from build123d import *

# Parameters (mm, degrees)
BOSS_EXTRUDE1_DEPTH = 1
SKETCH2_R           = 1
SKETCH2_W           = 7
SKETCH2_H           = 23.92041254
SKETCH2_H_2         = 5
BOSS_EXTRUDE4_DEPTH = 29
BOSS_EXTRUDE5_DEPTH = 7
SKETCH2_4_R         = 1
CUT_EXTRUDE1_DEPTH  = 29
CUT_EXTRUDE2_REACH  = 70.069
SKETCH5_W           = 7
SKETCH5_H           = 2


with BuildPart() as part:
    # Sketch1 → Boss-Extrude1 (new body)
    with BuildSketch(Plane(origin=(0, 0, 0), x_dir=(1, 0, 0), z_dir=(0, 1, 0))):
        Polygon((46.188021535, 0), (23.094010768, 40), (-23.094010768, 40), (-46.188021535, 0), (-23.094010768, -40), (23.094010768, -40), align=None)
    extrude(amount=BOSS_EXTRUDE1_DEPTH)

    # Sketch2 → Boss-Extrude4 (add)
    # profile 1 of 5: a face of its own
    with BuildSketch(Plane(origin=(0, 1, 0), x_dir=(1, 0, 0), z_dir=(0, 1, 0))):
        with Locations(Location((-14.1, -4.8, 0), (0, 0, 90))):
            Circle(SKETCH2_R)
    # profile 2 of 5: a face of its own
    with BuildSketch(Plane(origin=(0, 1, 0), x_dir=(1, 0, 0), z_dir=(0, 1, 0))):
        with Locations(Location((-14.1, 4.8, 0), (0, 0, 90))):
            Circle(SKETCH2_R)
    # profile 3 of 5: a face of its own
    with BuildSketch(Plane(origin=(0, 1, 0), x_dir=(1, 0, 0), z_dir=(0, 1, 0))):
        with Locations((34.9, 0)):
            Rectangle(SKETCH2_W, SKETCH2_H)
        with Locations(Location((35.9, -4.8, 0), (0, 0, 90))):
            Circle(SKETCH2_R, mode=Mode.SUBTRACT)
        with Locations(Location((35.9, 4.8, 0), (0, 0, 90))):
            Circle(SKETCH2_R, mode=Mode.SUBTRACT)
    # profile 4 of 5: a face of its own
    with BuildSketch(Plane(origin=(0, 1, 0), x_dir=(1, 0, 0), z_dir=(0, 1, 0))):
        with Locations((-13.1, 9.46020627)):
            Rectangle(SKETCH2_W, SKETCH2_H_2)
    # profile 5 of 5: a face of its own
    with BuildSketch(Plane(origin=(0, 1, 0), x_dir=(1, 0, 0), z_dir=(0, 1, 0))):
        with Locations((-13.1, -9.46020627)):
            Rectangle(SKETCH2_W, SKETCH2_H_2)
    extrude(amount=BOSS_EXTRUDE4_DEPTH)

    # Sketch4 → Boss-Extrude5 (add)
    with BuildSketch(Plane.ZY.offset(16.6)):
        Polygon((-6.96020627, 10), (0, 20), (6.96020627, 10), (6.96020627, 30), (-6.96020627, 30), align=None)
    extrude(amount=-BOSS_EXTRUDE5_DEPTH)

    # Sketch2<4> → Cut-Extrude1 (cut)
    with BuildSketch(Plane(origin=(0, 1, 0), x_dir=(1, 0, 0), z_dir=(0, 1, 0))):
        with Locations(Location((-14.1, -4.8, 0), (0, 0, 90))):
            Circle(SKETCH2_4_R)
        with Locations(Location((-14.1, 4.8, 0), (0, 0, 90))):
            Circle(SKETCH2_4_R)
    extrude(amount=CUT_EXTRUDE1_DEPTH, mode=Mode.SUBTRACT)

    # Sketch5 → Cut-Extrude2 (cut, up to next)
    with BuildSketch(Plane(origin=(0, 30, 0), x_dir=(1, 0, 0), z_dir=(0, 1, 0)), mode=Mode.PRIVATE) as cut_extrude2_sk1:
        with Locations((-13.1, 0)):
            Rectangle(SKETCH5_W, SKETCH5_H)
    cut_extrude2_tool1 = extrude(cut_extrude2_sk1.sketch, amount=-CUT_EXTRUDE2_REACH, mode=Mode.PRIVATE) & part.part
    add(cut_extrude2_tool1.solids().sort_by_distance((-13.1, 30, 0))[0], mode=Mode.SUBTRACT)


solid = part.part
Input: part model. Units: mm. Frame: model coordinates. A direction names the side the tool comes from. Coordinates: 2 decimals unless noted, no trailing zeros. Loops run counter-clockwise (first coordinate to the right, second up) from the corner with the lowest first, then second, coordinate; pieces in that order, holes last. Notation, with made-up numbers: (-29, 40.25) -> (-9, 40.25) arc R28 cw to (-9, 58.25) -> close; hole circle Ø8 at (36, 1). An arc over 180 degrees is marked (long way). Write each question's results on one line, items separated by ' | '. Start each with the question number.
Q1. Section C-C, the plane z = 34. Return the cut outline in (x, y).
Q2. Pin query (flat end, axial travel): pin 1 (3.5 mm diameter, centred on x = -12.5, y = 22.5, fed in from -Z); pin 2 (0.6 mm diameter, centred on x = 35.5, z = 4.5, fed in from +Y); pin 3 (9 mm diameter, centred on y = 17, z = -8.5, fed in from +X). Return the tip coordinate at first contact, or that it passes through.
Q3. Section A-A, the plane y = 20. Return the cut outline in (x, z), plus the area to 3 significant figures.
Q4. Section B-B, the plane x = 8. Return the cut outline in (y, z).
Q5. Pull-direction query (Y, two-part tool) for faces 1 (the flat face through (-13, 15, -11.96)), 2 (the flat face through (-13, 5, 6.96)), 3 (the flat face through (-1, 0, -1)); classes: released by +Y, released by -Y, zero draft, split by the parting line, or undercut.
Q6. Reachability of faces 4 (the flat face through (-13, 5, -6.96)), 5 (the flat face through (-13, 24, -1)), 6 (the flat face through (35, 15, 11.96)) from +Z, -Z, +X, -X, +Y, -Y: full face, straight path, thin tool, end or side. Return the list, or none.
Q7. Ray query, line 1 (Z direction, x = 35.9, y = 7); line 2 (X direction, y = 20.25, z = 4.8); line 3 (Z direction, x = -14.1, y = 26.25). Return the intervals inside material, ascending. Write a range as from..to.
Found:
1) outline: (-26.56, 0) -> (26.56, 0) -> (26.56, 1) -> (-26.56, 1) -> close
2) pin 1: z = -11.96 | pin 2: y = 1 | pin 3: x = 38.4
3) outline: (-16.6, -11.96) -> (-9.6, -11.96) -> (-9.6, -1) -> (-16.6, -1) -> close; (-16.6, 1) -> (-9.6, 1) -> (-9.6, 11.96) -> (-16.6, 11.96) -> close; (31.4, -11.96) -> (38.4, -11.96) -> (38.4, 11.96) -> (31.4, 11.96) -> close; hole circle Ø2 at (-14.1, -4.8); hole circle Ø2 at (-14.1, 4.8); hole circle Ø2 at (35.9, -4.8); hole circle Ø2 at (35.9, 4.8) | area: 308 mm2
4) outline: (0, -40) -> (1, -40) -> (1, 40) -> (0, 40) -> close
5) face 1: zero draft | face 2: undercut | face 3: released by -Y
6) face 4: -X | face 5: -X, +Y | face 6: +Z, +X, -X, +Y
7) line 1: -11.96..-5.8, -3.8..3.8, 5.8..11.96 | line 2: -16.6..-15.1, -13.1..-9.6, 31.4..34.9, 36.9..38.4 | line 3: -11.96..-5.8, -3.8..-1, 1..3.8, 5.8..11.96
